Build history of the part. All positions in model axes, mm. A direction names the side the tool comes from. Give positions to 0.01 mm unless a question says otherwise; leave off trailing zeros. Write each loop counter-clockwise with the first axis right and the second up, starting at its lowest first coordinate (ties: lowest second). Pieces come first, ordered by that corner, then holes.
from build123d import *

# Parameters (mm, degrees)
SKETCH3_R          = 2.75
CUT_EXTRUDE2_DEPTH = 61.850225965
SKETCH4_W          = 19.5
SKETCH4_H          = 1.5


with BuildPart() as part:
    # Sketch2 → Revolve1 (revolve)
    with BuildSketch(Plane(origin=(0, 0, 0), x_dir=(1, 0, 0), z_dir=(0, 1, 0)), mode=Mode.PRIVATE) as revolve1_sk:
        Polygon((17.5, -7), (42.5, -7), (42.5, -2), (22.5, -2), (22.5, 2), (27.5, 2), (27.5, 9.5), (15.25, 9.5), (15.25, 7.5), (17.5, 7.5), align=None)
    revolve(revolve1_sk.sketch.rotate(Axis((0, 0, -30.507012698), (0, 0, 1)), 180), axis=Axis((0, 0, -30.507012698), (0, 0, 1)))

    # Sketch3 → Cut-Extrude2 (cut, through all)
    with BuildSketch(Plane.XY):
        with Locations((0, 37.5)):
            Circle(SKETCH3_R)
        with Locations((37.5, 0)):
            Circle(SKETCH3_R)
        with Locations((0, -37.5)):
            Circle(SKETCH3_R)
        with Locations((-37.5, 0)):
            Circle(SKETCH3_R)
    extrude(amount=CUT_EXTRUDE2_DEPTH, mode=Mode.SUBTRACT)

    # Sketch4 → Cut-Revolve1 (revolve, cut)
    with BuildSketch(Plane(origin=(0, 0, 0), x_dir=(1, 0, 0), z_dir=(0, 1, 0)), mode=Mode.PRIVATE) as cut_revolve1_sk:
        with Locations((9.75, -4.25)):
            Rectangle(SKETCH4_W, SKETCH4_H)
    revolve(cut_revolve1_sk.sketch.rotate(Axis((0, 0, -30.507012698), (0, 0, 1)), 180), axis=Axis((0, 0, -30.507012698), (0, 0, 1)), mode=Mode.SUBTRACT)


solid = part.part
1. Drop flat-ended pins along their axis: pin 1 (5 mm diameter, centred on y = 3.5, z = 3.5, fed in from -X); pin 2 (7 mm diameter, centred on x = 37.5, y = 0, fed in from -Z); pin 3 (10.5 mm diameter, centred on x = -7.5, y = -3.5, fed in from +Z); pin 4 (9 mm diameter, centred on x = 0, y = -37.5, fed in from +Z). Give the stop position or say it passes through.
2. 3-axis set-ups, long thin cutter, end or side, ignore diameter. For faces 1 (the face through (-40.247, 0.121, 4.465)), 2 (the face through (-10.382, 19.961, -0.028)), 3 (the face through (3.794, 17.084, -1.923)): which of +Z, -Z, +X, -X, +Y, -Y reach the whole face in a straight line?
3. Saw through at C-C on z = -5.25. Give the cut face in (x, y).
4. Saw through at A-A on x = -37.5. Give the cut face in (y, z), plus the area to 4 significant figures.
5. Saw through at D-D on x = 0. Count the separate pieces of the cut face and the enclosed holes in it, plus the area to 3 significant figures.
6. Drill centre lines: line 1 along Y through (x, z) = (0, 4.5); line 2 along Z through (x, y) = (6, 17.5); line 3 along Y through (x, z) = (0, -4). Where is each one in solid material? Low to high.
7. Mould opens along Z. For faces 4 (the face through (-1, 18, 7)), 5 (the face through (-13, -12, 3.5)), 6 (the face through (-12.69, 24.397, -5.802)), 7 (the face through (-23, 0, -2)) say: pulls with the +Z half, pulls with the -Z half, needs draft (parallel to the pull), parting line crosses it, or undercut.
Outcome:
1. pin 1: stops at x = -42.49
1. pin 2: stops at z = 2
1. pin 3: passes through
1. pin 4: stops at z = 7
2. face 1: +Z, -Z
2. face 2: none
2. face 3: +Z
3. outline: circle Ø55 at (0, 0); hole circle Ø35 at (0, 0)
4. outline: (-20, 2) - (-2.75, 2) - (-2.75, 7) - (-20, 7) - close; (2.75, 2) - (20, 2) - (20, 7) - (2.75, 7) - close
4. area: 172.5 mm2
5. separate pieces: 4
5. enclosed holes: 0
5. area: 388 mm2
6. line 1: y = -42.5 to -40.25, -34.75 to -19.5, 19.5 to 34.75, 40.25 to 42.5
6. line 2: z = -9.5 to 3.5, 5 to 7
6. line 3: y = -27.5 to -17.5, 17.5 to 27.5
7. face 4: pulls with the +Z half
7. face 5: undercut
7. face 6: needs draft
7. face 7: undercut
